from build123d import *

# Parameters (mm, degrees)
F0_W     = 50.8
F0_H     = 19.05
F1_DEPTH = 774.7
F2_W     = 122.43557321
F2_H     = 50.8
F2_W_2   = 343.1604206562
F3_DEPTH = 25.4
F4_R     = 4.7625
F5_DEPTH = 25.4


# Not quite as in the source:
# - a feature names something its author has since deleted; it is built from what else it names


with BuildPart() as f1:
    # F0 (on Top) → F1 (new body)
    with BuildSketch(Plane.XY):
        Rectangle(F0_W, F0_H)
    extrude(amount=F1_DEPTH)

    # F2 (on Front) → F3 (cut)
    with BuildSketch(Plane.XZ):
        with Locations((22.4465244144, 25.4)):
            Rectangle(F2_W, F2_H)
        with Locations((-38.7818217278, 749.3)):
            Rectangle(F2_W_2, F2_H)
    extrude(amount=F3_DEPTH, mode=Mode.SUBTRACT)

    # F4 (on Front) → F5 (cut)
    with BuildSketch(Plane.XZ):
        with Locations((0, 25.4)):
            Circle(F4_R)
    extrude(amount=-F5_DEPTH, mode=Mode.SUBTRACT)


solid = f1.part
The model under review builds one solid part; all positions refer to its coordinate system, in mm. A direction names the side the tool comes from. Round coordinates to 2 decimals unless told otherwise and drop trailing zeros. Order: outer loops, then holes, each group sorted by start corner. A loop starts at its lowest first (then second) coordinate and runs counter-clockwise, first axis right, second up. Notation, with made-up numbers: (-30, 62) -> (26, 62) arc R18 cw to (26, 67) -> close; hole circle Ø1 at (40, -24.5). An arc over 180 degrees is marked (long way). Use CSV: the item, a comma, the result in double quotes. Start each with the question number.
(1) Insertion check: pin 1 (5 mm diameter, centred on x = -9, y = -6.5, fed in from +Z); pin 2 (15 mm diameter, centred on x = -2.5, z = 748.5, fed in from -Y); pin 3 (3 mm diameter, centred on x = -11.5, y = -6.5, fed in from -Z). Each pin has a flat end and moves straight along its axis. Give the tip position at first contact, or say it passes through.
(2) Consider section B-B on y = -5. Write out the cut boundary in (x, z), and give its area (3 significant figures).
(3) Tool access review of faces 1 (the face through (0, 0, 750)), 2 (the face through (-25.4, 0, 382)), 3 (the face through (5, 0, 26)): name each direction out of +Z, -Z, +X, -X, +Y, -Y from which nothing blocks a thin tool from reaching the whole face with its end or side.
(4) Wall thickness on probe 1 along Z at (x, y) = (0, 2); probe 2 along Z at (x, y) = (-1, 4.75); probe 3 along Z at (x, y) = (6.5, -5): over which ranges is each line inside the solid? List them lowest first. Write a range as from..to.
(5) Consider section A-A on x = -15.5. Write out the cut boundary in (y, z) (3 decimals), and give its area (3 significant figures).
Responses:
1,pin 1,"z = 723.9"
1,pin 2,"y = 0"
1,pin 3,"z = 50.8"
2,outline,"(-25.4, 50.8) -> (25.4, 50.8) -> (25.4, 723.9) -> (-25.4, 723.9) -> close"
2,area,"34,200 mm²"
3,face 1,"+Z, +X, -X, -Y"
3,face 2,"+Z, -Z, -X, +Y, -Y"
3,face 3,"-Z, +X, -X, -Y"
4,probe 1,"0..20.64, 30.16..774.7"
4,probe 2,"0..20.74, 30.06..774.7"
4,probe 3,"50.8..723.9"
5,outline,"(-9.525, 50.8) -> (0, 50.8) -> (0, 0) -> (9.525, 0) -> (9.525, 774.7) -> (0, 774.7) -> (0, 723.9) -> (-9.525, 723.9) -> close"
5,area,"13,800 mm²"
